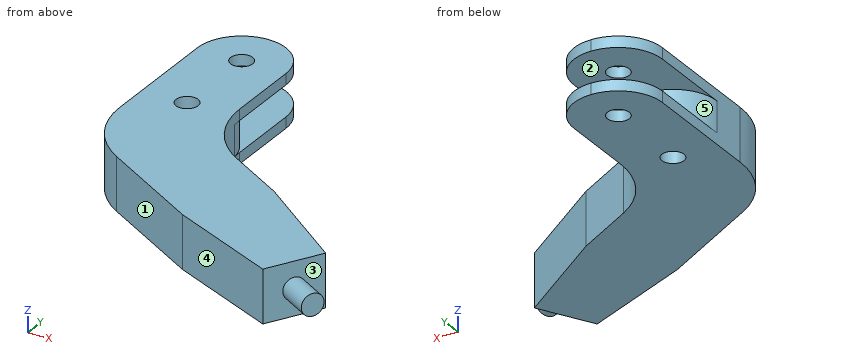
Autodesk Inventor part; units mm, degrees
ref_plane "YZ Plane" through (0, 0, 0) normal (1, 0, 0) x (0, 1, 0)
ref_plane "XZ Plane" through (0, 0, 0) normal (0, 1, 0) x (-1, 0, 0)
ref_plane "XY Plane" through (0, 0, 0) normal (0, 0, 1) x (1, 0, 0)
sketch "スケッチ1" plane through (0, 0, 0) normal (0, 0, 1) x (1, 0, 0)
  line L0 (0, 0) -> (40, 0)
  line L1 (40, 0) -> (40, 318)
  line L2 (40, 318) -> (0, 318)
  line L3 (0, 318) -> (0, 0)
  line L4 (0, 218) -> (112.7627, 152.8964)
  line L5 (112.7627, 152.8964) -> (132.7627, 187.5375)
  line L6 (132.7627, 187.5375) -> (40, 241.094)
  point P0 (40, 218)
  point P1 (40, 194.906)
  point P2 (20, 318)
  point P3 (122.7627, 170.2169)
  dimension "d0" = 40
  dimension "d1" = 318
  dimension "d69" = 40
  dimension "d70" = 60
  dimension "d91" = 20
  dimension "d92" = 100
  dimension "d93" = 180
extrude "押し出し1" add sketch "スケッチ1" along normal blind 24 contours L3 L2 L1 L4 | L1 L6 L5 L4
sketch "スケッチ6" plane through (0, 0, 24) normal (0, 0, 1) x (1, 0, 0)
  circle A0 centre (20, 258) radius 5
  line L0 (40, 318) -> (0, 318)
  line L1 (40, 241.094) -> (40, 318)
  circle A1 centre (20, 20) radius 1.2295
  circle A2 centre (20, 10) radius 1.2295
  line L2 (0, 0) -> (40, 0)
  circle A3 centre (20, 298) radius 5
  point P0 (20, 318)
  point P1 (40, 190.8114)
  point P2 (30, 0)
  dimension "d42" = 10
  dimension "d44" = 20
  dimension "d45" = 2.459
  dimension "d46" = 2.459
  dimension "d47" = 10
  dimension "d48" = 10
  dimension "d49" = 20
  dimension "d50" = 20
  dimension "d53" = 10
  dimension "d54" = 20
  dimension "d55" = 40
  dimension "d56" = 20
extrude "押し出し4" cut sketch "スケッチ6" against normal through all
sketch "スケッチ8" plane through (0, 0, 0) normal (-1, 0, 0) x (0, 0, 1)
  line L0 (0, 318) -> (24, 318)
  line L1 (5, 318) -> (19, 318)
  line L2 (19, 318) -> (19, 278)
  line L3 (19, 278) -> (5, 278)
  line L4 (5, 278) -> (5, 318)
  line L5 (0, 318) -> (0, 0)
  dimension "d57" = 5
  dimension "d58" = 14
  dimension "d59" = 40
extrude "押し出し5" cut sketch "スケッチ8" against normal through all
fillet "フィレット1" radius 20 4 edges at (40, 318, 21.5) (40, 318, 2.5) (0, 318, 2.5) (0, 318, 21.5)
fillet "フィレット2" radius 40 2 edges at (0, 218, 12) (40, 241.094, 12)
sketch "スケッチ9" plane through (0, 0, 24) normal (0, 0, 1) x (1, 0, 0)
  line L0 (20, 206.453) -> (112.7627, 152.8964)
  line L1 (132.7627, 187.5375) -> (60, 229.547)
  line L2 (112.7627, 152.8964) -> (132.7627, 187.5375)
  line L3 (132.7627, 187.5375) -> (112.7627, 152.8964)
  line L4 (66.3813, 179.6747) -> (112.7627, 152.8964)
  line L5 (132.7627, 187.5375) -> (166.773, 167.9016)
  line L6 (115.1204, 126.9801) -> (133.5174, 158.8446)
  line L7 (141.7531, 173.1092) -> (128.7627, 180.6092)
  line L8 (112.7627, 152.8964) -> (20, 206.453)
  line L9 (132.7627, 187.5375) -> (60, 229.547)
  line L10 (115.1204, 126.9801) -> (125.7531, 145.3964)
  line L11 (133.5174, 158.8446) -> (145.7531, 180.0375)
  line L12 (116.7627, 159.8246) -> (129.7531, 152.3246)
  line L13 (66.3813, 179.6747) -> (129.7531, 152.3246)
  line L14 (66.3813, 179.6747) -> (86.3813, 214.3157)
  line L15 (86.3813, 214.3157) -> (141.7531, 173.1092)
  point P0 (0, 0)
  point P1 (254.4532, 80.329)
  point P2 (128.7627, 180.6092)
  point P3 (123.2579, 156.0746)
  point P4 (86.3813, 214.3157)
  point P5 (40, 194.906)
  point P6 (115.8875, 158.3088)
  point P7 (129.6379, 182.1251)
  dimension "d80" = 24
  dimension "d81" = 40
  dimension "d83" = 15
  dimension "d84" = 8
  dimension "d90" = 24
extrude "押し出し6" cut sketch "スケッチ9" against normal through all contours L13 L2 L0 | L1 L2 L15
sketch "スケッチ11" plane through (104.9897, 139.4332, 24) normal (0.8660254, -0.5, 0) x (0, 0, -1)
  line L0 (0, 21.7957) -> (0, 49.2964)
  line L1 (24, 21.7957) -> (24, 49.2964)
  line L2 (0, 24) -> (24, 24)
  line L3 (24, 24) -> (24, 0)
  line L4 (24, 0) -> (0, 0)
  line L5 (0, 0) -> (0, 24)
  line L6 (17, 17) -> (7, 17)
  line L7 (7, 17) -> (7, 7)
  line L8 (7, 7) -> (17, 7)
  line L9 (17, 7) -> (17, 17)
  line L10 (0, 35.546) -> (24, 35.546)
  circle A0 centre (12, 35.546) radius 5
  point P0 (24, -173.2475)
  point P1 (24, 24)
  point P2 (0, 15.546)
  point P3 (0, 55.546)
  point P4 (24, 15.546)
  point P5 (24, 55.546)
  dimension "d85" = 10
  dimension "d88" = 10
extrude "押し出し7" add sketch "スケッチ11" along normal blind 15 contours A0 L10 | L10 A0
fillet "フィレット4" radius 20 2 edges at (0, 278, 12) (40, 278, 12)
equation "\"d45\" = d46"
equation "\"d48\" = d47"
equation "\"d50\" = d49"
properties part number "l_r_k2a__legparts_06(six)"
Design review of the part built by this model. Coordinates are the model's own, in mm. Face numbers are marked on the shaded views. A direction names the side the tool comes from. Give positions to 0.01 mm unless a question says otherwise; leave off trailing zeros. Order: outer loops, then holes, each group sorted by start corner. A loop starts at its lowest first (then second) coordinate and runs counter-clockwise, first axis right, second up. Notation, with made-up numbers: (19, 53.25) - (56, 53.25) arc R7 cw to (56, 61.25) - close; hole circle Ø11 at (0, -22). An arc over 180 degrees is marked (long way). Write item = value, one per line. Start each with the question number.
Q1. Tool access review of the marked faces 4 and 5: name each direction out of +Z, -Z, +X, -X, +Y, -Y from which nothing blocks a thin tool from reaching the whole face with its end or side.
Q2. To check wall thickness, follow L1, parallel to Y at x = 20, z = 3.45; L2, parallel to X at y = 298, z = 2.5; L3, parallel to Z at x = 14.5, y = 307. State the ranges of each line that lie inside material, in increasing order. Write a range as from..to.
Q3. We need section B-B on z = 2.25. State how many separate pieces and enclosed holes the cut face has, plus the area to 3 significant figures.
Q4. Clearance check with flat-ended pins moving along their axes: pin 1 Ø1.5 at (y, z) = (275.5, 22) entering from +X; pin 2 Ø3 at (x, z) = (15, 12) entering from +Y; pin 3 Ø6 at (x, y) = (20, 298) entering from +Z; pin 4 Ø1 at (x, z) = (112, 12) entering from +Y. State where each tip first meets the part, or that it passes through.
Q5. Mouldability with a two-part tool opening along X and no side actions: class the marked faces 1, 2 and 3 as released by +X, released by -X, zero draft, split by the parting line, or undercut.
Q6. We need section C-C on y = 198.5. State the section outline as (x, z) points.
Q7. We need section A-A on y = 286. State the section outline as (x, z) points.
Q8. We need section D-D on x = 99.5. State the section outline as (y, z) points.
Working result:
q1.face_4 = +Z, -Z, -X, -Y
q1.face_5 = -X, +Y
q2.L1 = 206.45..253, 263..293, 303..318
q2.L2 = 0..15, 25..40
q2.L3 = 0..5, 19..24
q3.separate_pieces = 1
q3.enclosed_holes = 2
q3.area = 7,620 mm²
q4.pin_1 = 40
q4.pin_2 = 277.69
q4.pin_3 = through
q4.pin_4 = 195.62
q5.face_1 = released by -X
q5.face_2 = zero draft
q5.face_3 = undercut
q6.outline = (33.77, 0) - (107.63, 0) - (107.63, 24) - (33.77, 24) - close
q7.outline = (0, 0) - (40, 0) - (40, 5) - (0, 5) - close; (0, 19) - (40, 19) - (40, 24) - (0, 24) - close
q8.outline = (165.38, 0) - (204.55, 0) - (204.55, 24) - (165.38, 24) - close
